Model file for the job. Use its own axes, mm. A direction names the side the tool comes from. Round coordinates to 2 decimals unless told otherwise and drop trailing zeros. Loops run counter-clockwise (first coordinate to the right, second up) from the corner with the lowest first, then second, coordinate; pieces in that order, holes last. Notation, with made-up numbers: (-2, -2) -> (18, -2) arc R28 ccw to (18, 18) -> close; hole circle Ø10 at (65, 78.5). An arc over 180 degrees is marked (long way). Use a Markdown table: item, result. Add a question column.
```python
from build123d import *

# Parameters (mm, degrees)
SKETCH1_W           = 65.6
SKETCH1_H           = 20
BOSS_EXTRUDE1_DEPTH = 4
SKETCH2_W           = 67
SKETCH2_H           = 90
BOSS_EXTRUDE2_DEPTH = 4
SKETCH3_R           = 0.8
CUT_EXTRUDE2_DEPTH  = 4
SKETCH4_R           = 0.8
CUT_EXTRUDE4_DEPTH  = 3.5


with BuildPart() as part:
    # Sketch1 → Boss-Extrude1 (new body)
    with BuildSketch(Plane.XY.offset(28)):
        with Locations((-118.3, 0)):
            Rectangle(SKETCH1_W, SKETCH1_H)
    extrude(amount=BOSS_EXTRUDE1_DEPTH)

    # Sketch2 → Boss-Extrude2 (add)
    with BuildSketch(Plane(origin=(-151.1, 0, 0), x_dir=(0, 0, -1), z_dir=(1, 0, 0))):
        with Locations((1.5, 0)):
            Rectangle(SKETCH2_W, SKETCH2_H)
    extrude(amount=BOSS_EXTRUDE2_DEPTH)

    # Sketch3 → Cut-Extrude2 (cut)
    with BuildSketch(Plane.XY.offset(28)):
        with Locations((-109.3, 4.5)):
            Circle(SKETCH3_R)
        with Locations((-109.3, -4.5)):
            Circle(SKETCH3_R)
        with Locations((-118.3, 4.5)):
            Circle(SKETCH3_R)
        with Locations((-118.3, -4.5)):
            Circle(SKETCH3_R)
    extrude(amount=CUT_EXTRUDE2_DEPTH, mode=Mode.SUBTRACT)

    # Sketch4 → Cut-Extrude4 (cut)
    with BuildSketch(Plane(origin=(-151.1, 0, 0), x_dir=(0, 0, -1), z_dir=(1, 0, 0))):
        with Locations((15, -30)):
            Circle(SKETCH4_R)
        with Locations((-15, -30)):
            Circle(SKETCH4_R)
        with Locations((15, 30)):
            Circle(SKETCH4_R)
        with Locations((-15, 30)):
            Circle(SKETCH4_R)
    extrude(amount=CUT_EXTRUDE4_DEPTH, mode=Mode.SUBTRACT)


solid = part.part
```
1) Tool access for faces 1 (the face through (-149, -45, -1)), 2 (the face through (-117, -10, 30)), 3 (the face through (-117, 10, 30)), 4 (the face through (-151.1, 1, -1)), 5 (the face through (-117, 0, 28)): list every direction of +Z, -Z, +X, -X, +Y, -Y with a clear straight run to the whole face (end or side of a thin tool).
2) Wall check: probe 1 along Y at (x, z) = (-118.3, 30.85); probe 2 along Y at (x, z) = (-149.15, 15); probe 3 along X at (y, z) = (-4, 30). Give the ranges that are in metal, low to high. Write a range as from..to.
3) Pin check, flat tips, straight feed: pin 1 Ø8 at (y, z) = (-27, -10.5) entering from +X; pin 2 Ø8 at (x, y) = (-134.5, 7.5) entering from -Z; pin 3 Ø0.5 at (y, z) = (-30, 14.5) entering from -X; pin 4 Ø1.4 at (x, y) = (-109.3, -4.5) entering from -Z. Stop position of each tip, or through.
4) Cut at C-C on x = -93.5. Write the cut outline in (y, z).
5) Cut at B-B on z = 8.5. Write the cut outline in (x, y).
6) Cut at A-A on y = -1.5. Write the cut outline in (x, z), and give its area (3 significant figures).
Established:
| question | item | result |
|---|---|---|
| 1 | face 1 | +Z, -Z, +X, -X, -Y |
| 1 | face 2 | +Z, -Z, +X, -Y |
| 1 | face 3 | +Z, -Z, +X, +Y |
| 1 | face 4 | +Z, -Z, -X, +Y, -Y |
| 1 | face 5 | -Z, +X, +Y, -Y |
| 2 | probe 1 | y = -10..-5.3, -3.7..3.7, 5.3..10 |
| 2 | probe 2 | y = -45..-30.8, -29.2..29.2, 30.8..45 |
| 2 | probe 3 | x = -151.1..-118.92, -117.68..-109.92, -108.68..-85.5 |
| 3 | pin 1 | stops at x = -147.1 |
| 3 | pin 2 | stops at z = 28 |
| 3 | pin 3 | stops at x = -147.6 |
| 3 | pin 4 | passes through |
| 4 | outline | (-10, 28) -> (10, 28) -> (10, 32) -> (-10, 32) -> close |
| 5 | outline | (-151.1, -45) -> (-147.1, -45) -> (-147.1, 45) -> (-151.1, 45) -> close |
| 6 | outline | (-151.1, -35) -> (-147.1, -35) -> (-147.1, 28) -> (-85.5, 28) -> (-85.5, 32) -> (-151.1, 32) -> close |
| 6 | area | 514 mm^2 |
